from build123d import *

# Parameters (mm, degrees)
SKETCH1_W           = 80
SKETCH1_H           = 80
BOSS_EXTRUDE1_DEPTH = 2
SKETCH4_R           = 1.5
CUT_EXTRUDE3_DEPTH  = 114.154761279
SKETCH6_R           = 1.5
CUT_EXTRUDE4_DEPTH  = 114.154761279
SKETCH8_R           = 20
SKETCH8_R_2         = 1.5
CUT_EXTRUDE6_DEPTH  = 114.154761279


with BuildPart() as part:
    # Sketch1 → Boss-Extrude1 (new body)
    with BuildSketch(Plane(origin=(0, 0, 0), x_dir=(1, 0, 0), z_dir=(0, 1, 0))):
        with Locations((40, 40)):
            Rectangle(SKETCH1_W, SKETCH1_H)
    extrude(amount=BOSS_EXTRUDE1_DEPTH)

    # Sketch4 → Cut-Extrude3 (cut, through all)
    with BuildSketch(Plane.XZ):
        with Locations(Location((5, -5, 0), (0, 0, 270))):
            Circle(SKETCH4_R)
        with Locations(Location((75, -5, 0), (0, 0, 90))):
            Circle(SKETCH4_R)
        with Locations(Location((75, -75, 0), (0, 0, 270))):
            Circle(SKETCH4_R)
        with Locations(Location((5, -75, 0), (0, 0, 90))):
            Circle(SKETCH4_R)
    extrude(amount=-CUT_EXTRUDE3_DEPTH, mode=Mode.SUBTRACT)

    # Sketch6 → Cut-Extrude4 (cut, through all)
    with BuildSketch(Plane(origin=(0, 2, 0), x_dir=(1, 0, 0), z_dir=(0, 1, 0))):
        with Locations(Location((8, 17.2, 0), (0, 0, 270))):
            Circle(SKETCH6_R)
        with Locations(Location((72, 17.2, 0), (0, 0, 270))):
            Circle(SKETCH6_R)
    cut_extrude4 = extrude(amount=-CUT_EXTRUDE4_DEPTH, mode=Mode.SUBTRACT)

    # Mirror1: Cut-Extrude4 across plane
    add(cut_extrude4.mirror(Plane.XY.offset(-40)), mode=Mode.SUBTRACT)

    # Sketch8 → Cut-Extrude6 (cut, through all)
    with BuildSketch(Plane(origin=(0, 2, 0), x_dir=(1, 0, 0), z_dir=(0, 1, 0))):
        with Locations(Location((40, 40, 0), (0, 0, 270))):
            Circle(SKETCH8_R)
        with Locations(Location((40, 72.5, 0), (0, 0, 270))):
            Circle(SKETCH8_R_2)
        with Locations(Location((72.5, 40, 0), (0, 0, 270))):
            Circle(SKETCH8_R_2)
        with Locations(Location((40, 7.5, 0), (0, 0, 270))):
            Circle(SKETCH8_R_2)
        with Locations(Location((7.5, 40, 0), (0, 0, 270))):
            Circle(SKETCH8_R_2)
    extrude(amount=-CUT_EXTRUDE6_DEPTH, mode=Mode.SUBTRACT)


solid = part.part
Here's how the part is built. I have some questions about the finished solid (model axes, mm). Coordinates: 2 decimals unless noted, no trailing zeros. Order: outer loops, then holes, each group sorted by start corner. A loop starts at its lowest first (then second) coordinate and runs counter-clockwise, first axis right, second up. Notation, with made-up numbers: M -12,26 L 20,26 A27 ccw 20,50 Z; hole C -27.5,-27 d9. An arc over 180 degrees is marked long. Answer as CSV lines item,"result".
Item 1: Imagine slicing it at A-A on z = -5. Write out the boundary of the cut face in (x, y), plus the area to 3 significant figures.
Results found:
outline,"M 0,0 L 3.5,0 L 3.5,2 L 0,2 Z; M 6.5,0 L 73.5,0 L 73.5,2 L 6.5,2 Z; M 76.5,0 L 80,0 L 80,2 L 76.5,2 Z"
area,"148 mm2"
Item 2: If I drill on line 1 (X direction, y = 1.2, z = -17.2); line 2 (Z direction, x = 75, y = 1.4); line 3 (X direction, y = 0.6, z = -5), over which ranges is the centre line in solid material (lowest first)?
Results found:
line 1,"0 to 6.5, 9.5 to 70.5, 73.5 to 80"
line 2,"-80 to -76.5, -73.5 to -6.5, -3.5 to 0"
line 3,"0 to 3.5, 6.5 to 73.5, 76.5 to 80"
Item 3: For pin 1 (4 mm diameter, centred on x = 75, z = -5, fed in from -Y); pin 2 (2.5 mm diameter, centred on x = 5, z = -5, fed in from +Y), each with a flat end and sliding along its axis, tell me the tip position at first contact or that it passes through.
Results found:
pin 1,"y = 0"
pin 2,"through"
Item 4: Imagine slicing it at C-C on z = -40. Write out the boundary of the cut face in (x, y), plus the area to 3 significant figures.
Results found:
outline,"M 0,0 L 6,0 L 6,2 L 0,2 Z; M 9,0 L 20,0 L 20,2 L 9,2 Z; M 60,0 L 71,0 L 71,2 L 60,2 Z; M 74,0 L 80,0 L 80,2 L 74,2 Z"
area,"68.0 mm2"
Item 5: Imagine slicing it at B-B on x = 40. Write out the boundary of the cut face in (y, z).
Results found:
outline,"M 0,-80 L 2,-80 L 2,-74 L 0,-74 Z; M 0,-71 L 2,-71 L 2,-60 L 0,-60 Z; M 0,-20 L 2,-20 L 2,-9 L 0,-9 Z; M 0,-6 L 2,-6 L 2,0 L 0,0 Z"
Item 6: We'd pull the mould along Z, two halves only. Please class faces 1 (the face through (38.536, 1.014, -7.825)), 2 (the face through (39, 1, -80)), 3 (the face through (0, 1, -39)): +Z half, -Z half, draft (parallel to the pull), parting line (faces both ways), or undercut.
Results found:
face 1,"undercut"
face 2,"-Z half"
face 3,"draft"
Item 7: Imagine slicing it at D-D on x = 75. Write out the boundary of the cut face in (y, z), plus the area to 3 significant figures.
Results found:
outline,"M 0,-80 L 2,-80 L 2,-76.5 L 0,-76.5 Z; M 0,-73.5 L 2,-73.5 L 2,-6.5 L 0,-6.5 Z; M 0,-3.5 L 2,-3.5 L 2,0 L 0,0 Z"
area,"148 mm2"
